Source: CAD feature listing. Evaluate the final solid. Frame: model axes, mm. Face numbers are marked on the shaded views. Give positions to 0.01 mm unless a question says otherwise; leave off trailing zeros. Write each loop counter-clockwise with the first axis right and the second up, starting at its lowest first coordinate (ties: lowest second). Pieces come first, ordered by that corner, then holes. Notation, with made-up numbers: (-13, -39.75) -> (26, -39.75) arc R23 ccw to (26, -12.75) -> close; hole circle Ø2 at (-9, -9). An arc over 180 degrees is marked (long way). Answer as a JSON object with one key per item and string values. Group by question number.
Item 1: Ray query, probe 1 along Y at (x, z) = (0, -7.75); probe 2 along Y at (x, z) = (0, -5.25); probe 3 along Z at (x, y) = (-16.5, -21.5). Return the intervals inside material, ascending. Write a range as from..to.
Item 2: Section query B-B on z = -14.75. Return the cut outline in (x, y), plus the area to 3 significant figures.
Item 3: Section query A-A on y = 0. Return the cut outline in (x, z), plus the area to 3 significant figures.
Item 4: First-contact query: pin 1 Ø1.6 at (x, z) = (-28.5, -9.5) entering from -Y; pin 2 Ø1.6 at (y, z) = (29, -8) entering from +X; pin 3 Ø1.5 at (y, z) = (-11.5, -11.5) entering from +X; pin 4 Ø8 at (x, y) = (-18.5, -19.5) entering from +Z. Flat tips, straight axial feed; report the tip coordinate or a pass-through.
Item 5: Pull-direction query (X, two-part tool) for the marked faces 1 and 2; classes: pulls with the +X half, pulls with the -X half, needs draft (parallel to the pull), parting line crosses it, or undercut.
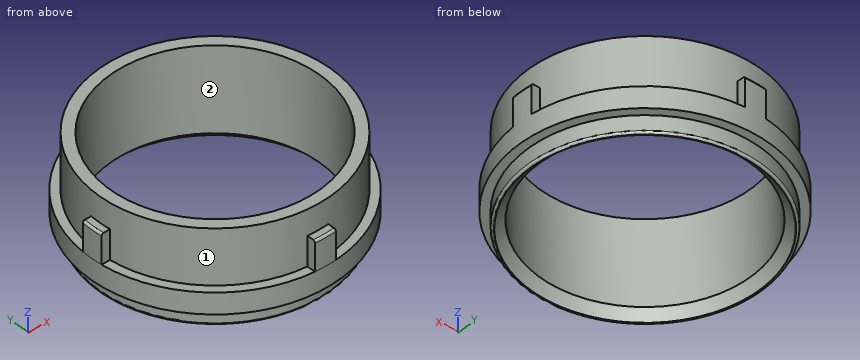
from build123d import *

# Parameters (mm, degrees)
F2_R            = 0.5
F3_SIZE         = 2
F5_DEPTH        = 7
F5_COPIES_COUNT = 4
F6_R            = 0.5


# Not quite as in the source:
# - after a boolean that leaves OpenCascade's solid faulty, fix() repairs it
# - a pattern or mirror of a feature is missing from the dataset's text; its kind, count and spacing are read off the source's solid


with BuildPart() as f1:
    # F0 (on Front) → F1 (revolve)
    with BuildSketch(Plane.XZ):
        Polygon((27.5, 0), (24.85, 0), (24.85, -22), (27.5, -22), (27.5, -18), (29.5, -18), (29.5, -13), (27.5, -13), align=None)
    revolve(axis=Axis((0, 0, -6.1865765601), (0, 0, -1)))

    # F2
    f2_edges = [f1.edges().sort_by_distance(p)[0] for p in [
        (-27.5, 0, -22),
    ]]
    fillet(f2_edges, radius=F2_R)

    # F3
    f3_edges = [f1.edges().sort_by_distance(p)[0] for p in [
        (-24.85, 0, -22),
    ]]
    chamfer(f3_edges, length=F3_SIZE)

    # F4 (on face) → F5 (join)
    with BuildSketch(Plane.XY.offset(-13)):
        with BuildLine():
            Line((-2.5, 29.3938769134), (-2.5, 27.3861278753))
            Line((-2.5, 27.3861278753), (2.5, 27.3861278753))
            Line((2.5, 27.3861278753), (2.5, 29.3938769134))
            ThreePointArc((2.5, 29.3938769134), (0, 29.5), (-2.5, 29.3938769134))
        make_face()
    f5 = extrude(amount=F5_DEPTH)

    # F5_copies: F5 ×4 about axis
    f5_copies_axis = Axis((0, 0, 0), (0, 0, 1))
    for i in range(1, F5_COPIES_COUNT):
        add(f5.rotate(f5_copies_axis, i * 360 / F5_COPIES_COUNT))

    add(f1.part.fix(), mode=Mode.REPLACE)

    # F6
    f6_edges = [f1.edges().sort_by_distance(p)[0] for p in [
        (0, 29.5, -6),
        (-29.5, 0, -6),
        (0, -29.5, -6),
        (29.5, 0, -6),
    ]]
    fillet(f6_edges, radius=F6_R)


solid = f1.part
Worked answers:
{
 "1": {"probe 1": "-29.5..-24.85, 24.85..29.5", "probe 2": "-27.5..-24.85, 24.85..27.5", "probe 3": "-21.99..0"},
 "2": {"outline": "circle Ø59 at (0, 0); hole circle Ø49.7 at (0, 0)", "area": "794 mm^2"},
 "3": {"outline": "(-29.5, -18) -> (-27.5, -18) -> (-27.5, -21.5) arc R0.5 ccw to (-27, -22) -> (-26.85, -22) -> (-24.85, -20) -> (-24.85, 0) -> (-27.5, 0) -> (-27.5, -6) -> (-29, -6) arc R0.5 ccw to (-29.5, -6.5) -> close; (24.85, -20) -> (26.85, -22) -> (27, -22) arc R0.5 ccw to (27.5, -21.5) -> (27.5, -18) -> (29.5, -18) -> (29.5, -6.5) arc R0.5 ccw to (29, -6) -> (27.5, -6) -> (27.5, 0) -> (24.85, 0) -> close", "area": "160 mm^2"},
 "4": {"pin 1": "y = -2.5", "pin 2": "x = 2.5", "pin 3": "x = 25.31", "pin 4": "z = 0"},
 "5": {"face 1": "parting line crosses it", "face 2": "undercut"}
}
